Part model, mm, in its own coordinate system. A direction names the side the tool comes from. Give positions to 0.01 mm unless a question says otherwise; leave off trailing zeros. Write each loop counter-clockwise with the first axis right and the second up, starting at its lowest first coordinate (ties: lowest second). Pieces come first, ordered by that corner, then holes. Notation, with made-up numbers: M 11.25,10 L 41.25,10 A17 cw 41.25,41 Z; hole C 63,-16.5 d5. An arc over 180 degrees is marked long. Answer as CSV lines item,"result". Start each with the question number.
Item 1: Band-saw the part on A-A, the plane x = -61.5. List the corners of the cut face in (y, z).
Item 2: Wall check: L1, parallel to X at y = 2.1, z = -3.5; L2, parallel to Z at x = -61.5, y = -8.3; L3, parallel to X at y = 9, z = -14.5. Give the ranges that are in metal, low to high. Write a range as from..to.
Item 3: Two-plate mould, pull along Z, no slides. Class faces 4 (the flat face through (-33, 1, -35)), 5 (the cylindrical face through (-4.886, -8.521, -30.925)), 6 (the flat face through (-65, -4, -17)): +Z half, -Z half, draft (parallel to the pull), parting line (faces both ways), or undercut.
Item 4: Pin check, flat tips, straight feed: pin 1 (2.5 mm diameter, centred on x = -39.5, y = 2, fed in from +Z); pin 2 (4 mm diameter, centred on x = -61.5, z = -31.5, fed in from +Y); pin 3 (10 mm diameter, centred on x = -47, y = 9.5, fed in from +Z); pin 4 (4 mm diameter, centred on x = -3.5, z = -31.5, fed in from -Y). Stop position of each tip, or through.
Item 5: Band-saw the part on C-C, the plane z = 2. List the corners of the cut face in (x, y).
Item 6: 3-axis set-ups, long thin cutter, end or side, ignore diameter. For faces 1 (the flat face through (-32, -9, 0)), 2 (the flat face through (-32, -7, -17)), 3 (the flat face through (-32, -10, -17)): which of +Z, -Z, +X, -X, +Y, -Y reach the whole face in a straight line?
Item 7: Band-saw the part on D-D, the plane z = -17.5. List the corners of the cut face in (x, y), then the cut area to 3 significant figures.
Item 8: Band-saw the part on B-B, the plane y = 12.5. List the corners of the cut face in (x, z), then the cut area to 3 significant figures.
Autodesk Inventor part; units mm, degrees
ref_plane "Work Plane1" through (0, 1.5, 0) normal (0, 1, 0) x (-1, 0, 0)
ref_plane "Work Plane2" through (-65, -7, 0) normal (1, 0, 0) x (0, 1, 0)
ref_plane "Work Plane3" through (0, 0, 0) normal (1, 0, 0) x (0, 1, 0)
sketch "Sketch2" plane through (0, 0, 0) normal (0, 1, 0) x (-1, 0, 0)
  line L0 (0, 0) -> (65, 0)
  line L1 (65, 0) -> (65, -35)
  line L2 (65, -35) -> (0, -35)
  line L3 (0, -35) -> (0, 0)
  dimension "d1" = 65
  dimension "d2" = 35
extrude "Extrusion1" add sketch "Sketch2" along normal blind 3
ref_plane "Work Plane1" through (0, 1.5, 0) normal (0, 1, 0) x (-1, 0, 0)
sketch "Sketch5" plane through (0, 0, 0) normal (0, 1, 0) x (-1, 0, 0)
  circle A0 centre (3.5, -31.5) radius 1.5
  circle A1 centre (3.5, -3.5) radius 1.5
  circle A2 centre (61.5, -31.5) radius 1.5
  circle A3 centre (61.5, -3.5) radius 1.5
  line L0 (0, 0) -> (0, -35)
  line L1 (65, -35) -> (65, 0)
  line L2 (0, -35) -> (65, -35)
  line L3 (65, 0) -> (0, 0)
  dimension "d22" = 3
  dimension "d23" = 3
  dimension "d24" = 3
  dimension "d25" = 3
  dimension "d26" = 3.5
  dimension "d27" = 3.5
  dimension "d28" = 3.5
  dimension "d29" = 3.5
  dimension "d30" = 3.5
  dimension "d31" = 3.5
  dimension "d32" = 3.5
  dimension "d33" = 3.5
extrude "Extrusion4" cut sketch "Sketch5" along normal blind 10 contours A0 | A1 | A2 | A3
pattern_linear "Rectangular Pattern1" count 2 spacing 10 along (0, -1, 0)
ref_plane "Work Plane2" through (-65, -7, 0) normal (1, 0, 0) x (0, 1, 0)
sketch "Sketch6" plane through (-65, -7, 0) normal (1, 0, 0) x (0, 1, 0)
  line L0 (7, -35) -> (10, -35)
  line L1 (-3, -35) -> (0, -35)
  line L2 (-3, 0) -> (0, 0)
  circle A0 centre (3.5, -17.5) radius 23
  line L3 (-3, -35) -> (-3, 0)
  line L4 (10, -35) -> (10, 0)
  point P0 (7, 0)
  point P1 (8.5, -35)
  point P2 (-1.5, -35)
  point P3 (-1.5, 0)
  point P4 (-1.5, -35)
extrude "Extrusion5" add sketch "Sketch6" against normal blind 3
ref_plane "Work Plane3" through (0, 0, 0) normal (1, 0, 0) x (0, 1, 0)
sketch "Sketch7" plane through (0, 0, 0) normal (1, 0, 0) x (0, 1, 0)
  circle A0 centre (-3.5, -17.5) radius 23
  line L0 (-10, 0) -> (-10, -35)
  line L1 (3, 0) -> (3, -35)
  line L2 (0, 0) -> (3, 0)
  line L3 (-10, -35) -> (-7, -35)
  dimension "d49" = 46
extrude "Extrusion6" add sketch "Sketch7" along normal blind 3
equation "\"d26\" = d27"
equation "\"d29\" = d28"
equation "\"d30\" = d28"
equation "\"d31\" = d27"
equation "\"d32\" = d26"
equation "\"d33\" = d30"
properties part number "koszyk na elektro"
Output:
1,outline,"M -10,-35 L -7,-35 L -7,-33 L -10,-33 Z; M -10,-30 L -7,-30 L -7,-5 L -10,-5 Z; M -10,-2 L -7,-2 L -7,0 L -10,0 Z; M 0,-35 L 3,-35 L 3,-33 L 0,-33 Z; M 0,-30 L 3,-30 L 3,-5 L 0,-5 Z; M 0,-2 L 3,-2 L 3,0 L 0,0 Z"
2,L1,"-68..-63, -60..-5, -2..3"
2,L2,"-35..-33, -30..-5, -2..0"
2,L3,"-68..-65, 0..3"
3,face 4,"-Z half"
3,face 5,"undercut"
3,face 6,"draft"
4,pin 1,"z = 0"
4,pin 2,"y = 3"
4,pin 3,"through"
4,pin 4,"y = -10"
5,outline,"M -68,-15.7 L -65,-15.7 L -65,8.7 L -68,8.7 Z; M 0,-15.7 L 3,-15.7 L 3,8.7 L 0,8.7 Z"
6,face 1,"+Z, +Y, -Y"
6,face 2,"+Z, -Z"
6,face 3,"+Z, -Z, -Y"
7,outline,"M -68,-26.5 L -65,-26.5 L -65,-10 L 0,-10 L 0,-26.5 L 3,-26.5 L 3,19.5 L 0,19.5 L 0,3 L -65,3 L -65,19.5 L -68,19.5 Z; hole M -65,-7 L 0,-7 L 0,0 L -65,0 Z"
7,area,"666 mm²"
8,outline,"M -68,-34.02 L -65,-34.02 L -65,-0.98 L -68,-0.98 Z; M 0,-34.02 L 3,-34.02 L 3,-0.98 L 0,-0.98 Z"
8,area,"198 mm²"
